```python
from build123d import *

# Parameters (mm, degrees)
F1_DEPTH = 670
F2_R     = 4
F3_R     = 2.4
F4_W     = 37
F4_H     = 35.4
F5_DEPTH = 4
F6_R     = 3
F7_DEPTH = 25


with BuildPart() as f1:
    # F0 (on Right) → F1 (new body, symmetric)
    with BuildSketch(Plane.YZ):
        Polygon((-146.6, 0), (145, 0), (145, -31.4), (146.6, -31.4), (146.6, 1.6), (-145, 1.6), (-145, 33), (-146.6, 33), align=None)
    extrude(amount=F1_DEPTH, both=True)

    # F2
    f2_edges = [f1.edges().sort_by_distance(p)[0] for p in [
        (0, -146.6, 0),
        (0, 146.6, 1.6),
    ]]
    fillet(f2_edges, radius=F2_R)

    # F3
    f3_edges = [f1.edges().sort_by_distance(p)[0] for p in [
        (0, -145, 1.6),
        (0, 145, 0),
    ]]
    fillet(f3_edges, radius=F3_R)

    # F4 (on face) → F5 (cut)
    with BuildSketch(Plane(origin=(0, 146.6, 0), x_dir=(-1, 0, 0), z_dir=(0, 1, 0))):
        with Locations((-651.5, -13.7)):
            Rectangle(F4_W, F4_H)
        with Locations((651.5, -13.7)):
            Rectangle(F4_W, F4_H)
    extrude(amount=-F5_DEPTH, mode=Mode.SUBTRACT)

    # F6 (on face) → F7 (cut)
    with BuildSketch(Plane.XY.offset(1.6)):
        with Locations((-647, -46.6)):
            Circle(F6_R)
        with Locations((-647, 53.4)):
            Circle(F6_R)
        with Locations((647, 53.4)):
            Circle(F6_R)
        with Locations((647, -46.6)):
            Circle(F6_R)
    extrude(amount=-F7_DEPTH, mode=Mode.SUBTRACT)


solid = f1.part
```
Geometry: final body of the model. Coordinates: model frame, mm. A direction names the side the tool comes from. Round coordinates to 2 decimals unless told otherwise and drop trailing zeros. Write each loop counter-clockwise with the first axis right and the second up, starting at its lowest first coordinate (ties: lowest second). Pieces come first, ordered by that corner, then holes. Notation, with made-up numbers: (67, -13) -> (116, -13) arc R30 ccw to (116, 14) -> close; hole circle Ø10 at (67.5, 10). An arc over 180 degrees is marked (long way). Use CSV: the item, a comma, the result in double quotes. Start each with the question number.
Q1. Section A-A (x = 448). Return loops of the section in (y, z), plus the area to 3 significant figures.
Q2. Reachability of faces 1 (the face through (9, -2, 0)), 2 (the face through (9, 2, 1.6)), 3 (the face through (9, 146.6, -17)) from +Z, -Z, +X, -X, +Y, -Y: full face, straight path, thin tool, end or side. Return the list, or none.
Q3. Section B-B (y = 79). Return loops of the section in (x, z), plus the area to 3 significant figures.
Q4. First-contact query: pin 1 Ø0.5 at (x, z) = (-644.5, 1) entering from +Y; pin 2 Ø1 at (x, z) = (-12.5, 25.5) entering from +Y; pin 3 Ø8 at (x, y) = (-40.5, 100.5) entering from -Z; pin 4 Ø5.5 at (x, y) = (-647, -46.6) entering from -Z. Flat tips, straight axial feed; report the tip coordinate or a pass-through.
Q5. Line query: L1, parallel to Y at x = 647, z = 0.9; L2, parallel to Y at x = -647, z = 1; L3, parallel to X at y = 53, z = 1. Output: solid intervals per line, ascending.
Q6. Section C-C (z = -20). Return loops of the section in (x, y).
Result sheet:
1,outline,"(-146.6, 4) arc R4 ccw to (-142.6, 0) -> (142.6, 0) arc R2.4 cw to (145, -2.4) -> (145, -31.4) -> (146.6, -31.4) -> (146.6, -2.4) arc R4 ccw to (142.6, 1.6) -> (-142.6, 1.6) arc R2.4 cw to (-145, 4) -> (-145, 33) -> (-146.6, 33) -> close"
1,area,"565 mm²"
2,face 1,"-Z, +X, -X, -Y"
2,face 2,"+Z, +X, -X, +Y"
2,face 3,"+Z, -Z, +X, -X, +Y"
3,outline,"(-670, 0) -> (670, 0) -> (670, 1.6) -> (-670, 1.6) -> close"
3,area,"2,140 mm²"
4,pin 1,"y = 142.6"
4,pin 2,"y = -145"
4,pin 3,"z = 0"
4,pin 4,"through"
5,L1,"-145.13 to -49.6, -43.6 to 50.4, 56.4 to 142.6"
5,L2,"-145.25 to -49.6, -43.6 to 50.4, 56.4 to 142.6"
5,L3,"-670 to -649.97, -644.03 to 644.03, 649.97 to 670"
6,outline,"(-633, 145) -> (633, 145) -> (633, 146.6) -> (-633, 146.6) -> close"
